Answer from the drawing. Dimensions are ordinates in mm from the lowest x, y and z of the part. Round coordinates to 2 decimals unless told otherwise and drop trailing zeros. Order: outer loops, then holes, each group sorted by start corner. A loop starts at its lowest first (then second) coordinate and runs counter-clockwise, first axis right, second up. Notation, with made-up numbers: (45.5, 19.5) - (75.5, 19.5) arc R14 cw to (75.5, 31.5) - close; hole circle Ø1 at (52, 23). An arc over 180 degrees is marked (long way). One line per question, with ' | ' between items. Start each with the question number.
1) The part is cut by section C-C, the plane y = 0.7. Count the separate pieces of the cut face and the enclosed holes in it, plus the area to 3 significant figures.
2) The part is cut by section A-A, the plane x = 15. Give the vertices of the cut face in (y, z).
3) The part is cut by section B-B, the plane z = 59. Give the vertices of the cut face in (x, y).
4) Straight lines are drawn through the part: line 1 (X direction, y = 0.85, z = 59); line 2 (Z direction, x = 105, y = 0.7); line 3 (Z direction, x = 110, y = 1.95). For each, find the intervals that lie inside material, in ascending order. Write a range as from..to.
5) Flat-ended cylindrical pins translate along their axes: pin 1 (3 mm diameter, centred on x = 65, z = 65.5, fed in from +Y); pin 2 (4 mm diameter, centred on x = 105, z = 25.5, fed in from -Y). Find the tip coordinate at first contact, or state that the pin passes through.
6) The part is cut by section D-D, the plane x = 42. Give the vertices of the cut face in (y, z), plus the area to 3 significant figures.
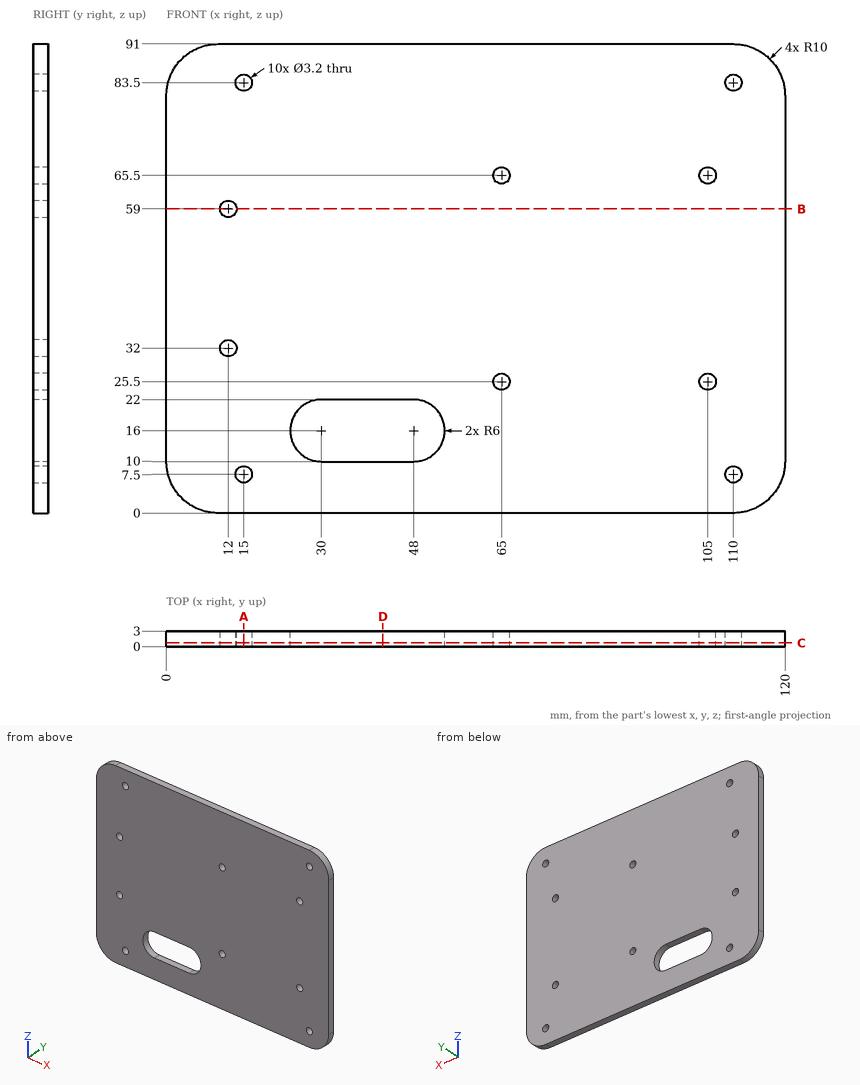
Values:
1) separate pieces: 1 | enclosed holes: 11 | area: 10,400 mm^2
2) outline: (0, 0) - (3, 0) - (3, 5.9) - (0, 5.9) - close; (0, 9.1) - (3, 9.1) - (3, 81.9) - (0, 81.9) - close; (0, 85.1) - (3, 85.1) - (3, 91) - (0, 91) - close
3) outline: (0, 0) - (10.4, 0) - (10.4, 3) - (0, 3) - close; (13.6, 0) - (120, 0) - (120, 3) - (13.6, 3) - close
4) line 1: x = 0..10.4, 13.6..120 | line 2: z = 0..23.9, 27.1..63.9, 67.1..91 | line 3: z = 0..5.9, 9.1..81.9, 85.1..91
5) pin 1: passes through | pin 2: stops at y = 0
6) outline: (0, 0) - (3, 0) - (3, 10) - (0, 10) - close; (0, 22) - (3, 22) - (3, 91) - (0, 91) - close | area: 237 mm^2
